Design review of the part built by this model. Coordinates are the model's own, in mm. A direction names the side the tool comes from. Give positions to 0.01 mm unless a question says otherwise; leave off trailing zeros. Write each loop counter-clockwise with the first axis right and the second up, starting at its lowest first coordinate (ties: lowest second). Pieces come first, ordered by that corner, then holes. Notation, with made-up numbers: (7.25, 25.5) -> (57.25, 25.5) arc R27 cw to (57.25, 44.5) -> close; hole circle Ø9 at (-5, 36.5). An arc over 180 degrees is marked (long way). Answer as a JSON object with one key per item and string values.
```python
from build123d import *

# Parameters (mm, degrees)
F1_DEPTH = 6.35


with BuildPart() as f1:
    # F0 (on Front) → F1 (new body)
    with BuildSketch(Plane.XZ):
        Polygon((-13.9372432471, -7.1591061907), (-6.593507121, -6.5868337818), (-9.6865712375, -1.1433150152), align=None)
        Polygon((-9.6865712375, -1.1433150152), (-6.593507121, -6.5868337818), (-0.8915456345, -9.172675501), (5.2413577367, -7.9131365257), (9.4626423545, -3.2893179343), (10.1599209711, 2.9326387291), (7.0668568545, 8.3761574957), (1.364895368, 10.9619992149), (-4.7680080032, 9.7024602396), (-8.989292621, 5.0786416482), align=None)
        Polygon((-0.8915456345, -9.172675501), (-6.593507121, -6.5868337818), (-6.4963796804, -13.9521933969), align=None)
        Polygon((-15.9641518481, 2.7102466722), (-9.6865712375, -1.1433150152), (-8.989292621, 5.0786416482), align=None)
        Polygon((5.2413577367, -7.9131365257), (-0.8915456345, -9.172675501), (3.5162818752, -15.0742865222), align=None)
        Polygon((-11.8028952898, 11.8861078451), (-8.989292621, 5.0786416482), (-4.7680080032, 9.7024602396), align=None)
        Polygon((9.4626423545, -3.2893179343), (5.2413577367, -7.9131365257), (12.2762450233, -10.0967841312), align=None)
        Polygon((-3.0429321417, 16.8636102361), (-4.7680080032, 9.7024602396), (1.364895368, 10.9619992149), align=None)
        Polygon((10.1599209711, 2.9326387291), (9.4626423545, -3.2893179343), (16.4375015816, -0.9209229583), align=None)
        Polygon((6.9697294139, 15.7415171108), (1.364895368, 10.9619992149), (7.0668568545, 8.3761574957), align=None)
        Polygon((7.0668568545, 8.3761574957), (10.1599209711, 2.9326387291), (14.4105929806, 8.9484299046), align=None)
    extrude(amount=F1_DEPTH)


solid = f1.part
```
(1) We need section A-A, the plane x = -13. State the section outline as (y, z) points, then the cut area to 3 significant figures.
Here are the results:
{"outline": "(-6.35, -7.09) -> (0, -7.09) -> (0, -5.83) -> (-6.35, -5.83) -> close; (-6.35, 0.89) -> (0, 0.89) -> (0, 3.72) -> (-6.35, 3.72) -> close", "area": "25.9 mm²"}
(2) Clearance check with a flat-ended pin moving along its axis: pin 1 (1.5 mm diameter, centred on x = 12, z = 10, fed in from -Y). State where the tip first meets the part, or that it passes through.
Here are the results:
{"pin 1": "passes through"}
(3) We need section D-D, the plane z = -2.5. State the section outline as (x, y) points, then the cut area to 3 significant figures.
Here are the results:
{"outline": "(-10.65, -6.35) -> (11.79, -6.35) -> (11.79, 0) -> (-10.65, 0) -> close", "area": "142 mm²"}
(4) The part is to be moulded in two halves that separate along Z. For faces 4 (the flat face through (0, 0, 1)), 5 (the flat face through (-12.43, -3.13, 3.91)), 6 (the flat face through (10.79, -3.131, 8.666)), say which applies: +Z half, -Z half, draft (parallel to the pull), parting line (faces both ways), or undercut.
Here are the results:
{"face 4": "draft", "face 5": "undercut", "face 6": "+Z half"}
(5) For line 1 along Z through (x, y) = (-12.5, -4.75); line 2 along X through (y, z) = (-2.25, 12.5); line 3 along Z through (x, y) = (-13.5, -4.5), list the stretches that pass through material, from the lowest coordinate up.
Here are the results:
{"line 1": "z = -7.05 to -5.13, 0.58 to 3.89", "line 2": "x = -4.09 to 0.22, 3.17 to 7.01", "line 3": "z = -7.13 to -6.54, 1.2 to 3.55"}
(6) For faces 1 (the flat face through (-3.9, -3.1, 13.3)), 2 (the flat face through (-10.317, -3.131, -6.877)), 3 (the flat face through (12.256, -3.131, 5.898)), list the 3-axis set-ups (+Z, -Z, +X, -X, +Y, -Y) from which the entire face can be reached by the end or side of a thin tool; tool diameter is ignored.
Here are the results:
{"face 1": "+Z, +Y, -Y", "face 2": "-Z, +Y, -Y", "face 3": "+X, +Y, -Y"}
(7) We need section B-B, the plane y = -3.5. State the section outline as (x, z) points, then the cut area to 3 significant figures.
Here are the results:
{"outline": "(-15.96, 2.71) -> (-9.69, -1.14) -> (-13.94, -7.16) -> (-6.59, -6.59) -> (-6.5, -13.95) -> (-0.89, -9.17) -> (3.52, -15.07) -> (5.24, -7.91) -> (12.28, -10.1) -> (9.46, -3.29) -> (16.44, -0.92) -> (10.16, 2.93) -> (14.41, 8.95) -> (7.07, 8.38) -> (6.97, 15.74) -> (1.36, 10.96) -> (-3.04, 16.86) -> (-4.77, 9.7) -> (-11.8, 11.89) -> (-8.99, 5.08) -> close", "area": "510 mm²"}
(8) We need section C-C, the plane x = 13.5. State the section outline as (y, z) points, then the cut area to 3 significant figures.
Here are the results:
{"outline": "(-6.35, -1.92) -> (0, -1.92) -> (0, 0.88) -> (-6.35, 0.88) -> close; (-6.35, 7.66) -> (0, 7.66) -> (0, 8.88) -> (-6.35, 8.88) -> close", "area": "25.5 mm²"}
